Work out the finished part from the listing and answer in its coordinate system (mm). Face numbers are marked on the shaded views. A direction names the side the tool comes from. Round coordinates to 2 decimals unless told otherwise and drop trailing zeros. Order: outer loops, then holes, each group sorted by start corner. A loop starts at its lowest first (then second) coordinate and runs counter-clockwise, first axis right, second up. Notation, with made-up numbers: (40.5, 32.25) - (51.5, 32.25) arc R16 cw to (51.5, 48.25) - close; hole circle Ø6 at (58, 85). An arc over 180 degrees is marked (long way). Answer in a Markdown table with one row per item.
Autodesk Fusion 360 part; units mm, degrees
sketch "Sketch1" plane through (0, 0, 0) normal (0, 0, 1) x (1, 0, 0)
  line L0 (25, 25) -> (67.5, 25)
  line L1 (67.5, 25) -> (67.5, 97)
  line L2 (67.5, 97) -> (25, 97)
  line L3 (25, 97) -> (25, 25)
  dimension "d1" = 42.5
  dimension "d2" = 72
extrude "Extrude1" add sketch "Sketch1" along normal blind 17.5
sketch "Sketch2" plane through (0, 0, 17.5) normal (0, 0, 1) x (-1, 0, 0)
  line L0 (-25, -97) -> (-25, -25)
  line L1 (-25, -25) -> (-67.5, -25)
  line L2 (-67.5, -25) -> (-67.5, -97)
  line L3 (-67.5, -97) -> (-25, -97)
  line L4 (-25, -97) -> (-26.5, -97)
  line L5 (-26.5, -97) -> (-26.5, -95.5)
  line L6 (-26.5, -95.5) -> (-25, -95.5)
  line L7 (-25, -95.5) -> (-25, -97)
  line L8 (-67.5, -25) -> (-66, -25)
  line L9 (-66, -25) -> (-66, -26.5)
  line L10 (-66, -26.5) -> (-67.5, -26.5)
  line L11 (-67.5, -26.5) -> (-67.5, -25)
  line L12 (-47, -25) -> (-45.5, -25) construction
  line L13 (-45.5, -25) -> (-45.5, -26.5) construction
  line L14 (-45.5, -26.5) -> (-47, -26.5) construction
  line L15 (-47, -26.5) -> (-47, -25) construction
  line L16 (-26.5, -95.5) -> (-45.5, -95.5)
  line L17 (-45.5, -95.5) -> (-45.5, -26.5)
  line L18 (-45.5, -26.5) -> (-26.5, -26.5)
  line L19 (-26.5, -26.5) -> (-26.5, -95.5)
  line L20 (-45.5, -97) -> (-47, -97)
  line L21 (-47, -97) -> (-47, -95.5)
  line L22 (-47, -95.5) -> (-45.5, -95.5)
  line L23 (-45.5, -95.5) -> (-45.5, -97)
  line L24 (-47, -95.5) -> (-66, -95.5)
  line L25 (-66, -95.5) -> (-66, -26.5)
  line L26 (-66, -26.5) -> (-47, -26.5)
  line L27 (-47, -26.5) -> (-47, -95.5)
  point P0 (-47, -25)
  point P1 (-45.5, -97)
  dimension "d5" = 1.5
  dimension "d6" = 1.5
  dimension "d7" = 1.5
  dimension "d8" = 1.5
  dimension "d9" = 22
  dimension "d10" = 1.5
  dimension "d11" = 1.5
  dimension "d12" = 22
  dimension "d15" = 1.5
  dimension "d16" = 1.5
extrude "Extrude2" cut sketch "Sketch2" against normal blind 16 contours L16 L17 L18 L19 | L24 L25 L26 L27
sketch "Sketch3" plane through (25, 0, 0) normal (-1, 0, 0) x (0, -1, 0)
  line L0 (-97, 0) -> (-25, 0)
  line L1 (-25, 0) -> (-25, 17.5)
  line L2 (-25, 17.5) -> (-97, 17.5)
  line L3 (-97, 17.5) -> (-97, 0)
  line L4 (-61, 0) -> (-61, 17.5) construction
  line L5 (-74, 5.5) -> (-48, 5.5)
  arc A0 (-48, 5.5) -> (-48, 29.5) centre (-48, 17.5) ccw
  line L6 (-48, 29.5) -> (-74, 29.5)
  arc A1 (-74, 29.5) -> (-74, 5.5) centre (-74, 17.5) ccw
  line L7 (-86, 17.5) -> (-36, 17.5) construction
  point P0 (-36, 17.5)
  point P1 (-86, 17.5)
  dimension "d19" = 25
  dimension "d20" = 25
  dimension "d21" = 24
extrude "Extrude3" cut sketch "Sketch3" against normal blind 42.5 contours L2 L5 A0 A1
fillet "Fillet1" radius 0.5 24 edges at (25, 39.5147, 9.0147) (25, 61, 5.5) (25, 82.4853, 9.0147) (45.5, 39.5147, 9.0147) (45.5, 61, 5.5) (45.5, 82.4853, 9.0147) (66, 39.5147, 9.0147) (66, 61, 5.5) (66, 82.4853, 9.0147) (26.5, 82.4853, 9.0147) (26.5, 61, 5.5) (26.5, 39.5147, 9.0147) (47, 82.4853, 9.0147) (47, 61, 5.5) (47, 39.5147, 9.0147) (67.5, 82.4853, 9.0147) (67.5, 61, 5.5) (67.5, 39.5147, 9.0147) (66.75, 36, 17.5) (46.25, 36, 17.5) (25.75, 36, 17.5) (25.75, 86, 17.5) (46.25, 86, 17.5) (66.75, 86, 17.5)
sketch "Sketch4" plane through (0, 0, 17.5) normal (0, 0, 1) x (-1, 0, 0)
  arc A0 (-67.4999, -86.49) -> (-67.5, -86.5) centre (-67, -86.5) ccw
  line L0 (-67.5, -86.5) -> (-67.5, -97)
  line L1 (-67.5, -97) -> (-25, -97)
  line L2 (-25, -97) -> (-25, -86.5)
  arc A1 (-25, -86.5) -> (-25.0001, -86.49) centre (-25.5, -86.5) ccw
  line L3 (-25.0001, -86.49) -> (-26.4999, -86.49)
  arc A2 (-26.4999, -86.49) -> (-26.5, -86.5) centre (-26, -86.5) ccw
  line L4 (-26.5, -86.5) -> (-26.5, -95.5)
  line L5 (-26.5, -95.5) -> (-45.5, -95.5)
  line L6 (-45.5, -95.5) -> (-45.5, -86.5)
  arc A3 (-45.5, -86.5) -> (-45.5001, -86.49) centre (-46, -86.5) ccw
  line L7 (-45.5001, -86.49) -> (-46.9999, -86.49)
  arc A4 (-46.9999, -86.49) -> (-47, -86.5) centre (-46.5, -86.5) ccw
  line L8 (-47, -86.5) -> (-47, -95.5)
  line L9 (-47, -95.5) -> (-66, -95.5)
  line L10 (-66, -95.5) -> (-66, -86.5)
  arc A5 (-66, -86.5) -> (-66.0001, -86.49) centre (-66.5, -86.5) ccw
  line L11 (-66.0001, -86.49) -> (-67.4999, -86.49)
  line L12 (-26.5, -95.5) -> (-25.5, -95.5)
  line L13 (-25.5, -95.5) -> (-25.5, -95.2)
  line L14 (-25.5, -95.2) -> (-26.5, -95.2)
  line L15 (-26.5, -95.2) -> (-26.5, -95.5)
  line L16 (-66, -95.5) -> (-67, -95.5)
  line L17 (-67, -95.5) -> (-67, -95.2)
  line L18 (-67, -95.2) -> (-66, -95.2)
  line L19 (-66, -95.2) -> (-66, -95.5)
  line L20 (-45.5, -95.5) -> (-46.15, -95.5)
  line L21 (-46.15, -95.5) -> (-46.15, -95.2)
  line L22 (-46.15, -95.2) -> (-45.5, -95.2)
  line L23 (-45.5, -95.2) -> (-45.5, -95.5)
  line L24 (-47, -95.5) -> (-46.35, -95.5)
  line L25 (-46.35, -95.5) -> (-46.35, -95.2)
  line L26 (-46.35, -95.2) -> (-47, -95.2)
  line L27 (-47, -95.2) -> (-47, -95.5)
  dimension "d25" = 1
  dimension "d26" = 0.3
  dimension "d27" = 1
  dimension "d28" = 0.3
  dimension "d29" = 0.65
  dimension "d30" = 0.3
  dimension "d42" = 0.65
  dimension "d43" = 0.3
sketch "Sketch5" plane through (0, 0, 17.5) normal (0, 0, 1) x (-1, 0, 0)
  arc A0 (-67.5, -35.5) -> (-67.4999, -35.51) centre (-67, -35.5) ccw
  line L0 (-67.4999, -35.51) -> (-66.0001, -35.51)
  arc A1 (-66.0001, -35.51) -> (-66, -35.5) centre (-66.5, -35.5) ccw
  line L1 (-66, -35.5) -> (-66, -26.5)
  line L2 (-66, -26.5) -> (-47, -26.5)
  line L3 (-47, -26.5) -> (-47, -35.5)
  arc A2 (-47, -35.5) -> (-46.9999, -35.51) centre (-46.5, -35.5) ccw
  line L4 (-46.9999, -35.51) -> (-45.5001, -35.51)
  arc A3 (-45.5001, -35.51) -> (-45.5, -35.5) centre (-46, -35.5) ccw
  line L5 (-45.5, -35.5) -> (-45.5, -26.5)
  line L6 (-45.5, -26.5) -> (-26.5, -26.5)
  line L7 (-26.5, -26.5) -> (-26.5, -35.5)
  arc A4 (-26.5, -35.5) -> (-26.4999, -35.51) centre (-26, -35.5) ccw
  line L8 (-26.4999, -35.51) -> (-25.0001, -35.51)
  arc A5 (-25.0001, -35.51) -> (-25, -35.5) centre (-25.5, -35.5) ccw
  line L9 (-25, -35.5) -> (-25, -25)
  line L10 (-25, -25) -> (-67.5, -25)
  line L11 (-67.5, -25) -> (-67.5, -35.5)
  line L12 (-26.5, -26.5) -> (-25.5, -26.5)
  line L13 (-25.5, -26.5) -> (-25.5, -26.8)
  line L14 (-25.5, -26.8) -> (-26.5, -26.8)
  line L15 (-26.5, -26.8) -> (-26.5, -26.5)
  line L16 (-45.5, -26.5) -> (-46.15, -26.5)
  line L17 (-46.15, -26.5) -> (-46.15, -26.8)
  line L18 (-46.15, -26.8) -> (-45.5, -26.8)
  line L19 (-45.5, -26.8) -> (-45.5, -26.5)
  line L20 (-47, -26.5) -> (-46.35, -26.5)
  line L21 (-46.35, -26.5) -> (-46.35, -26.8)
  line L22 (-46.35, -26.8) -> (-47, -26.8)
  line L23 (-47, -26.8) -> (-47, -26.5)
  line L24 (-66, -26.5) -> (-66.7, -26.5)
  line L25 (-66.7, -26.5) -> (-66.7, -26.8)
  line L26 (-66.7, -26.8) -> (-66, -26.8)
  line L27 (-66, -26.8) -> (-66, -26.5)
  dimension "d31" = 1
  dimension "d32" = 0.3
  dimension "d33" = 0.65
  dimension "d34" = 0.3
  dimension "d35" = 0.65
  dimension "d36" = 0.3
  dimension "d37" = 0.7
  dimension "d38" = 0.3
extrude "Extrude4" cut sketch "Sketch4" sketch "Sketch5" against normal blind 16 contours L10 L16 L17 L18 L19 | L8 L24 L25 L26 L27 | L4 L12 L13 L14 L15 | L6 L20 L21 L22 L23 of sketch 2 contours L1 L24 L25 L26 L27 | L3 L20 L21 L22 L23 | L7 L12 L13 L14 L15 | L5 L16 L17 L18 L19
fillet "Fillet2" radius 0.5 4 edges at (26.5, 61, 1.5) (45.5, 61, 1.5) (47, 61, 1.5) (66, 61, 1.5)
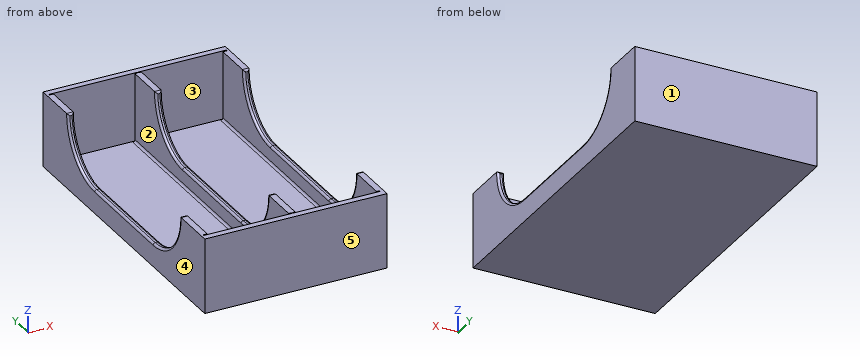
1) Find the intervals of material crossed by probe 1 along X at (y, z) = (92, 4.75); probe 2 along Y at (x, z) = (53, 2.75); probe 3 along Z at (x, y) = (37.5, 48), in increasing order. Write a range as from..to.
Filled in:
| item | result |
|---|---|
| probe 1 | x = 25..26.5, 45.5..47, 66..67.5 |
| probe 2 | y = 25..26.5, 95.5..97 |
| probe 3 | z = 0..1.5 |
2) Find section B-B, the plane x = 63.5. Give the vertices of the cut face in (y, z), then the cut area to 3 significant figures.
Filled in:
| item | result |
|---|---|
| outline | (25, 0) - (97, 0) - (97, 17.5) - (95.5, 17.5) - (95.5, 1.5) - (26.5, 1.5) - (26.5, 17.5) - (25, 17.5) - close |
| area | 156 mm^2 |
3) Each of these flat-tipped pins is pushed along its axis until it touches: pin 1 (0.6 mm diameter, centred on x = 67, y = 59.5, fed in from +Z); pin 2 (10.5 mm diameter, centred on x = 39, y = 58.5, fed in from +Z); pin 3 (1 mm diameter, centred on x = 29.5, y = 38.5, fed in from -Z); pin 4 (8 mm diameter, centred on y = 43, z = 15, fed in from -X). Where does it stop, or does it pass through?
Filled in:
| item | result |
|---|---|
| pin 1 | stops at z = 5.5 |
| pin 2 | stops at z = 1.5 |
| pin 3 | stops at z = 0 |
| pin 4 | passes through |
4) Find section A-A, the plane z = 3. Give the vertices of the cut face in (x, y), then the cut area to 3 significant figures.
Filled in:
| item | result |
|---|---|
| outline | (25, 25) - (67.5, 25) - (67.5, 97) - (25, 97) - close; hole (25.5, 26.5) - (46.15, 26.5) - (46.15, 26.8) - (45.5, 26.8) - (45.5, 95.2) - (46.15, 95.2) - (46.15, 95.5) - (25.5, 95.5) - (25.5, 95.2) - (26.5, 95.2) - (26.5, 26.8) - (25.5, 26.8) - close; hole (46.35, 26.5) - (66.7, 26.5) - (66.7, 26.8) - (66, 26.8) - (66, 95.2) - (67, 95.2) - (67, 95.5) - (46.35, 95.5) - (46.35, 95.2) - (47, 95.2) - (47, 26.8) - (46.35, 26.8) - close |
| area | 436 mm^2 |
5) Which of the six approach directions +Z, -Z, +X, -X, +Y, -Y give full straight-line access (tool end or side, diameter ignored) to the marked faces 1 and 2?
Filled in:
| item | result |
|---|---|
| face 1 | +Z, -Z, +X, -X, +Y |
| face 2 | +Z |
6) The mould has two halves that part along Y. Classify the marked faces 3, 4 and 5: released by +Y, released by -Y, zero draft, split by the parting line, or undercut.
Filled in:
| item | result |
|---|---|
| face 3 | undercut |
| face 4 | zero draft |
| face 5 | released by -Y |
7) Find section C-C, the plane y = 32. Give the vertices of the cut face in (x, z).
Filled in:
| item | result |
|---|---|
| outline | (25, 0) - (67.5, 0) - (67.5, 17.5) - (66, 17.5) - (66, 2) arc R0.5 cw to (65.5, 1.5) - (47.5, 1.5) arc R0.5 cw to (47, 2) - (47, 17.5) - (45.5, 17.5) - (45.5, 2) arc R0.5 cw to (45, 1.5) - (27, 1.5) arc R0.5 cw to (26.5, 2) - (26.5, 17.5) - (25, 17.5) - close |
8) Find section D-D, the plane y = 69.5. Give the vertices of the cut face in (x, z).
Filled in:
| item | result |
|---|---|
| outline | (25, 0) - (67.5, 0) - (67.5, 5) arc R0.5 ccw to (67, 5.5) - (66.5, 5.5) arc R0.5 ccw to (66, 5) - (66, 2) arc R0.5 cw to (65.5, 1.5) - (47.5, 1.5) arc R0.5 cw to (47, 2) - (47, 5) arc R0.5 ccw to (46.5, 5.5) - (46, 5.5) arc R0.5 ccw to (45.5, 5) - (45.5, 2) arc R0.5 cw to (45, 1.5) - (27, 1.5) arc R0.5 cw to (26.5, 2) - (26.5, 5) arc R0.5 ccw to (26, 5.5) - (25.5, 5.5) arc R0.5 ccw to (25, 5) - close |
